The model under review builds one solid part; all positions refer to its coordinate system, in mm. Face numbers are marked on the shaded views. A direction names the side the tool comes from. Coordinates: 2 decimals unless noted, no trailing zeros. Order: outer loops, then holes, each group sorted by start corner. A loop starts at its lowest first (then second) coordinate and runs counter-clockwise, first axis right, second up. Notation, with made-up numbers: M 72.25,-33.5 L 111.25,-33.5 A15 cw 111.25,-11.5 Z; hole C 80,89 d9. An arc over 180 degrees is marked long. One line per item, written item: value.
```python
from build123d import *

# Parameters (mm, degrees)
PAD_DEPTH       = 150
SKETCH001_W     = 17
SKETCH001_H     = 10
PAD001_DEPTH    = 25
SKETCH002_W     = 30
SKETCH002_H     = 60
PAD002_DEPTH    = 8
SKETCH003_W     = 13
SKETCH003_H     = 24
POCKET_DEPTH    = 8.001
SKETCH004_R     = 0.8
HOLE_DEPTH      = 25
CHAMFER_SIZE    = 16
CHAMFER001_SIZE = 3
PAD003_DEPTH    = 12
SKETCH006_W     = 15
SKETCH006_H     = 50
PAD004_DEPTH    = 10
SKETCH007_R     = 1.7
HOLE001_DEPTH   = 6
HOLE001_TIPS_R  = 1.7
SKETCH008_W     = 15
SKETCH008_H     = 50
PAD005_DEPTH    = 10
SKETCH009_R     = 1.7
HOLE002_DEPTH   = 6
HOLE002_TIPS_R  = 1.7
SKETCH010_W     = 15
SKETCH010_H     = 50
PAD006_DEPTH    = 10
SKETCH011_R     = 1.7
HOLE003_DEPTH   = 6
HOLE003_TIPS_R  = 1.7
SKETCH012_W     = 101
SKETCH012_H     = 15
PAD007_DEPTH    = 15
SKETCH013_W     = 12
SKETCH013_H     = 12
POCKET001_DEPTH = 151.501
SKETCH014_W     = 101
SKETCH014_H     = 15
PAD008_DEPTH    = 15
SKETCH015_W     = 12
SKETCH015_H     = 12
POCKET002_DEPTH = 190.7234318643


with BuildPart() as part:
    # Sketch → Pad (new body)
    with BuildSketch(Plane.XY):
        Polygon((87.4685657822, -50.5), (87.4685657822, 50.5), (0, 101), (-87.4685657822, 50.5), (-87.4685657822, -50.5), (0, -101), align=None)
        Polygon((86.6025403784, 50), (0, 100), (-86.6025403784, 50), (-86.6025403784, -50), (0, -100), (86.6025403784, -50), align=None, mode=Mode.SUBTRACT)
    extrude(amount=PAD_DEPTH)

    # Sketch001 (on Face13 of Pad) → Pad001 (join)
    with BuildSketch(Plane(origin=(0, 0, 0), x_dir=(1, 0, 0), z_dir=(0, 0, -1))):
        with Locations((95.1025403784, -5)):
            Rectangle(SKETCH001_W, SKETCH001_H)
    extrude(amount=PAD001_DEPTH)

    # Sketch002 (on Face20 of Pad001) → Pad002 (join)
    with BuildSketch(Plane(origin=(0, 0, -25), x_dir=(1, 0, 0), z_dir=(0, 0, -1))):
        with Locations((88.6025403784, 20)):
            Rectangle(SKETCH002_W, SKETCH002_H)
    extrude(amount=PAD002_DEPTH)

    # Sketch003 (on Face21 of Pad002) → Pocket (cut, through all)
    with BuildSketch(Plane.XY.offset(-25)):
        with Locations((82.6025403784, -20)):
            Rectangle(SKETCH003_W, SKETCH003_H)
    extrude(amount=-POCKET_DEPTH, mode=Mode.SUBTRACT)

    # Sketch004 (on Face21 of Pocket) → Hole (cut)
    with BuildSketch(Plane.XY.offset(-25)):
        with Locations((82.6025403784, -6.379604)):
            Circle(SKETCH004_R)
        with Locations((82.6025403784, -33.379604)):
            Circle(SKETCH004_R)
    extrude(amount=-HOLE_DEPTH, mode=Mode.SUBTRACT)

    # Chamfer
    chamfer_edges = [part.edges().sort_by_distance(p)[0] for p in [
        (87.468566, 5, 0),
    ]]
    chamfer(chamfer_edges, length=CHAMFER_SIZE)

    # Chamfer001
    chamfer001_edges = [part.edges().sort_by_distance(p)[0] for p in [
        (95.10254, 0, -25),
        (86.60254, 5, -25),
    ]]
    chamfer(chamfer001_edges, length=CHAMFER001_SIZE)

    # Sketch005 (on Face7 of Chamfer001) → Pad003 (join)
    with BuildSketch(Plane(origin=(0, 0, 0), x_dir=(1, 0, 0), z_dir=(0, 0, -1))):
        Polygon((86.6025403784, -10), (86.6025403784, -50), (0, -100), (-86.6025403784, -50), (-87.4685657822, -50.5), (0, -101), (87.4685657822, -50.5), (87.4685657822, -10), align=None)
    extrude(amount=PAD003_DEPTH)

    # Sketch006 (on Face23 of Pad003) → Pad004 (join)
    with BuildSketch(Plane.YZ.offset(87.4685657822)):
        with Locations((30.25, 13)):
            Rectangle(SKETCH006_W, SKETCH006_H)
    extrude(amount=PAD004_DEPTH)

    # Sketch007 (on Face47 of Pad004) → Hole001 (cut)
    with BuildSketch(Plane.YZ.offset(97.4685657822)):
        with Locations((30.25, 25.5)):
            Circle(SKETCH007_R)
        with Locations((30.25, 0.5)):
            Circle(SKETCH007_R)
    extrude(amount=-HOLE001_DEPTH, mode=Mode.SUBTRACT)

    # Hole001 tips → Hole001 tip 1 section 0
    with BuildSketch(Plane.YZ.offset(91.4685657822), mode=Mode.PRIVATE) as hole001_tip_1_s0:
        with Locations((30.25, 25.5)):
            Circle(HOLE001_TIPS_R)
    loft([hole001_tip_1_s0.sketch, Vertex(90.4471027299, 30.25, 25.5)], mode=Mode.SUBTRACT)

    # Hole001 tips → Hole001 tip 2 section 0
    with BuildSketch(Plane.YZ.offset(91.4685657822), mode=Mode.PRIVATE) as hole001_tip_2_s0:
        with Locations((30.25, 0.5)):
            Circle(HOLE001_TIPS_R)
    loft([hole001_tip_2_s0.sketch, Vertex(90.4471027299, 30.25, 0.5)], mode=Mode.SUBTRACT)

    # Sketch008 (on Face48 of Hole001) → Pad005 (join)
    with BuildSketch(Plane(origin=(43.7342828911, 75.75, 0), x_dir=(-0.8660254038, 0.5, 0), z_dir=(0.5, 0.8660254038, 0))):
        with Locations((0, 13)):
            Rectangle(SKETCH008_W, SKETCH008_H)
    extrude(amount=PAD005_DEPTH)

    # Sketch009 (on Face56 of Pad005) → Hole002 (cut)
    with BuildSketch(Plane(origin=(48.7342828911, 84.4102540378, 0), x_dir=(-0.8660254038, 0.5, 0), z_dir=(0.5, 0.8660254038, 0))):
        with Locations((0, 25.5)):
            Circle(SKETCH009_R)
        with Locations((0, 0.5)):
            Circle(SKETCH009_R)
    extrude(amount=-HOLE002_DEPTH, mode=Mode.SUBTRACT)

    # Hole002 tips → Hole002 tip 1 section 0
    with BuildSketch(Plane(origin=(45.7342828911, 79.2141016151, 0), x_dir=(-0.8660254038, 0.5, 0), z_dir=(0.5, 0.8660254038, 0)), mode=Mode.PRIVATE) as hole002_tip_1_s0:
        with Locations((0, 25.5)):
            Circle(HOLE002_TIPS_R)
    loft([hole002_tip_1_s0.sketch, Vertex(45.2235513649, 78.3294886628, 25.5)], mode=Mode.SUBTRACT)

    # Hole002 tips → Hole002 tip 2 section 0
    with BuildSketch(Plane(origin=(45.7342828911, 79.2141016151, 0), x_dir=(-0.8660254038, 0.5, 0), z_dir=(0.5, 0.8660254038, 0)), mode=Mode.PRIVATE) as hole002_tip_2_s0:
        with Locations((0, 0.5)):
            Circle(HOLE002_TIPS_R)
    loft([hole002_tip_2_s0.sketch, Vertex(45.2235513649, 78.3294886628, 0.5)], mode=Mode.SUBTRACT)

    # Sketch010 (on Face44 of Hole002) → Pad006 (join)
    with BuildSketch(Plane(origin=(-43.7342828911, 75.75, 0), x_dir=(-0.8660254038, -0.5, 0), z_dir=(-0.5, 0.8660254038, 0))):
        with Locations((0, 13)):
            Rectangle(SKETCH010_W, SKETCH010_H)
    extrude(amount=PAD006_DEPTH)

    # Sketch011 (on Face62 of Pad006) → Hole003 (cut)
    with BuildSketch(Plane(origin=(-48.7342828911, 84.4102540378, 0), x_dir=(-0.8660254038, -0.5, 0), z_dir=(-0.5, 0.8660254038, 0))):
        with Locations((0, 25.5)):
            Circle(SKETCH011_R)
        with Locations((0, 0.5)):
            Circle(SKETCH011_R)
    extrude(amount=-HOLE003_DEPTH, mode=Mode.SUBTRACT)

    # Hole003 tips → Hole003 tip 1 section 0
    with BuildSketch(Plane(origin=(-45.7342828911, 79.2141016151, 0), x_dir=(-0.8660254038, -0.5, 0), z_dir=(-0.5, 0.8660254038, 0)), mode=Mode.PRIVATE) as hole003_tip_1_s0:
        with Locations((0, 25.5)):
            Circle(HOLE003_TIPS_R)
    loft([hole003_tip_1_s0.sketch, Vertex(-45.2235513649, 78.3294886628, 25.5)], mode=Mode.SUBTRACT)

    # Hole003 tips → Hole003 tip 2 section 0
    with BuildSketch(Plane(origin=(-45.7342828911, 79.2141016151, 0), x_dir=(-0.8660254038, -0.5, 0), z_dir=(-0.5, 0.8660254038, 0)), mode=Mode.PRIVATE) as hole003_tip_2_s0:
        with Locations((0, 0.5)):
            Circle(HOLE003_TIPS_R)
    loft([hole003_tip_2_s0.sketch, Vertex(-45.2235513649, 78.3294886628, 0.5)], mode=Mode.SUBTRACT)

    # Sketch012 (on Face16 of Hole003) → Pad007 (join)
    with BuildSketch(Plane(origin=(-87.4685657822, 0, 0), x_dir=(0, -1, 0), z_dir=(-1, 0, 0))):
        with Locations((0, 47.5)):
            Rectangle(SKETCH012_W, SKETCH012_H)
    extrude(amount=PAD007_DEPTH)

    # Sketch013 (on Face61 of Pad007) → Pocket001 (cut, through all)
    with BuildSketch(Plane(origin=(0, 50.5, 0), x_dir=(-1, 0, 0), z_dir=(0, 1, 0))):
        with Locations((94.9685657822, 47.5)):
            Rectangle(SKETCH013_W, SKETCH013_H)
    extrude(amount=-POCKET001_DEPTH, mode=Mode.SUBTRACT)

    # Sketch014 (on Face27 of Pocket001) → Pad008 (join)
    with BuildSketch(Plane(origin=(43.7342828911, 75.75, 0), x_dir=(-0.8660254038, 0.5, 0), z_dir=(0.5, 0.8660254038, 0))):
        with Locations((0, 47.5)):
            Rectangle(SKETCH014_W, SKETCH014_H)
    extrude(amount=PAD008_DEPTH)

    # Sketch015 (on Face49 of Pad008) → Pocket002 (cut, through all)
    with BuildSketch(Plane(origin=(-43.7342828911, 25.25, 0), x_dir=(-0.5, -0.8660254038, 0), z_dir=(-0.8660254038, 0.5, 0))):
        with Locations((-94.9685657822, 47.5)):
            Rectangle(SKETCH015_W, SKETCH015_H)
    extrude(amount=-POCKET002_DEPTH, mode=Mode.SUBTRACT)


solid = part.part
```
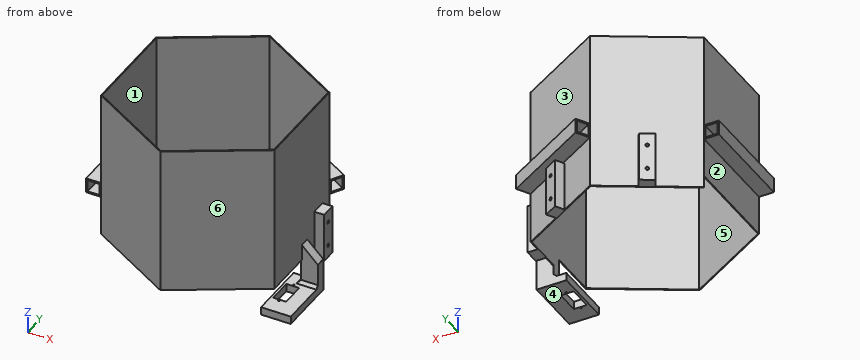
(1) Mouldability with a two-part tool opening along X and no side actions: class the marked faces 4, 5 and 6 as +X half, -X half, draft (parallel to the pull), parting line (faces both ways), or undercut.
Geometry results:
face 4: draft
face 5: undercut
face 6: +X half
(2) Tool access review of the marked faces 1, 2 and 3: name each direction out of +Z, -Z, +X, -X, +Y, -Y from which nothing blocks a thin tool from reaching the whole face with its end or side.
Geometry results:
face 1: +Z, -Z
face 2: -Z, -X, +Y, -Y
face 3: +Z, +X, +Y
(3) Insertion check: pin 1 Ø5 at (x, y) = (92.5, 30) entering from +Z; pin 2 Ø8 at (y, z) = (69, 129.5) entering from +X; pin 3 Ø11 at (x, z) = (94, 2.5) entering from +Y; pin 4 Ø7.5 at (x, z) = (-93, 48.5) entering from +Y. Each pin has a flat end and moves straight along its axis. Give the tip position at first contact, or say it passes through.
Geometry results:
pin 1: stops at z = 38
pin 2: stops at x = 62.35
pin 3: stops at y = 37.75
pin 4: passes through
(4) For L1, parallel to Z at x = 94, y = 30; L2, parallel to X at y = 28.5, z = 56; L3, parallel to Z at x = 83.5, y = -4.5, list the stretches that pass through material, from the lowest coordinate up.
Geometry results:
L1: z = -12 to -1.18, 2.18 to 23.82, 27.18 to 38
L2: x = -87.47 to -86.6, 86.6 to 87.47
L3: z = -33 to -25
(5) We need section C-C, the plane x = -11.5. State the section outline as (y, z) points, plus the area to 3 significant figures.
Geometry results:
outline: M -94.36,0 L -93.36,0 L -93.36,150 L -94.36,150 Z; M 93.36,-12 L 94.36,-12 L 94.36,150 L 93.36,150 Z
area: 312 mm2
(6) We need section D-D, the plane z = 82. State the section outline as (x, y) points.
Geometry results:
outline: M -87.47,-50.5 L 0,-101 L 87.47,-50.5 L 87.47,50.5 L 0,101 L -87.47,50.5 Z; hole M -86.6,-50 L 0,-100 L 86.6,-50 L 86.6,50 L 0,100 L -86.6,50 Z
(7) We need section A-A, the plane y = 19. State the section outline as (x, z) points, plus the area to 3 significant figures.
Geometry results:
outline: M -102.47,40 L -87.47,40 L -87.47,0 L -86.6,0 L -86.6,150 L -87.47,150 L -87.47,55 L -102.47,55 Z; M 86.6,-12 L 87.47,-12 L 87.47,150 L 86.6,150 Z; hole M -100.97,41.5 L -88.97,41.5 L -88.97,53.5 L -100.97,53.5 Z
area: 351 mm2
(8) We need section B-B, the plane z = 45.5. State the section outline as (x, y) points.
Geometry results:
outline: M -102.47,-50.5 L -100.97,-50.5 L -100.97,50.5 L -102.47,50.5 Z; M -88.97,-50.5 L -87.47,-50.5 L 0,-101 L 87.47,-50.5 L 87.47,50.5 L 88.22,51.8 L 0.75,102.3 L 0,101 L -87.47,50.5 L -88.97,50.5 Z; M 6.75,112.69 L 94.22,62.19 L 94.97,63.49 L 7.5,113.99 Z; hole M -86.6,-50 L 0,-100 L 86.6,-50 L 86.6,50 L 0,100 L -86.6,50 Z
